Part model, mm, in its own coordinate system. Give positions to 0.01 mm unless a question says otherwise; leave off trailing zeros. Write each loop counter-clockwise with the first axis right and the second up, starting at its lowest first coordinate (ties: lowest second). Pieces come first, ordered by that corner, then holes. Notation, with made-up numbers: M 14,57.25 L 24,57.25 A25 cw 24,91.25 Z; hole C 24,89.25 d11. An arc over 180 degrees is marked long. Answer as CSV lines item,"result". Start each with the question number.
Item 1: Band-saw the part on A-A, the plane y = 8. List the corners of the cut face in (x, z), then the cut area to 3 significant figures.
Item 2: Wall check: L1, parallel to X at y = 0.5, z = 23; L2, parallel to Z at x = 26.5, y = 0; L3, parallel to Z at x = 25, y = 2. Give the ranges that are in metal, low to high. Write a range as from..to.
Item 3: Pin check, flat tips, straight feed: pin 1 (8 mm diameter, centred on y = 0, z = -15, fed in from +X); pin 2 (4 mm diameter, centred on x = -21.5, y = 1, fed in from +Z); pin 3 (5.5 mm diameter, centred on y = 0.5, z = 17.5, fed in from -X). Stop position of each tip, or through.
Item 4: Band-saw the part on B-B, the plane y = 12.5. List the corners of the cut face in (x, z), then the cut area to 3 significant figures.
Item 5: Band-saw the part on C-C, the plane z = 29.5. Count the separate pieces of the cut face and the enclosed holes in it, then the cut area to 3 significant figures.
from build123d import *

# Parameters (mm, degrees)
REVOLVE1_ANGLE                 = 90
BOSS_EXTRUDE2_DEPTH            = 22.5
CUT_EXTRUDE1_DEPTH             = 57.762672959
MIRROR3_START                  = -2.736132077
MIRROR3_DEPTH                  = 5
MIRROR3_START_2                = 2.263867923
MIRROR3_2_DEPTH                = 20.236132077
MIRROR3_3_DEPTH                = 1
MIRROR3_START_3                = 1.263867923
MIRROR3_4_DEPTH                = 1
MIRROR4_START                  = -2.736132077
MIRROR4_DEPTH                  = 5
MIRROR4_START_2                = 2.263867923
MIRROR4_2_DEPTH                = 20.236132077
MIRROR4_3_DEPTH                = 1
MIRROR4_START_3                = 1.263867923
MIRROR4_4_DEPTH                = 1
SKETCH7_R                      = 3.35
CUT_EXTRUDE2_DEPTH             = 20
FILLET9_R                      = 0.5
CUT_EXTRUDE3_REACH             = 59.609
SKETCH8_R                      = 1.5
CUT_EXTRUDE3_DIRECTION_2_REACH = 59.609


# Read off the part's stored shape, not the designer's step: Mirror3, Mirror4
with BuildPart() as part:
    # Sketch1 → Revolve1 (revolve)
    with BuildSketch(Plane.XY):
        Polygon((0, 2.263867923), (0, -2.736132077), (37.5, -2.736132077), (37.5, -1.736132077), (37.25, -1.736132077), (37.25, 1.263867923), (37.5, 1.263867923), (37.5, 2.263867923), align=None)
    revolve(axis=Axis((0, 2.263867923, 0), (0, -1, 0)), revolution_arc=REVOLVE1_ANGLE)

    # Sketch2 → Boss-Extrude2 (add)
    with BuildSketch(Plane(origin=(0, 0, 0), x_dir=(1, 0, 0), z_dir=(0, 1, 0))):
        with BuildLine():
            Line((0, 0), (6, 0))
            ThreePointArc((6, 0), (4.242640687, -4.242640687), (0, -6))
            Line((0, -6), (0, 0))
        make_face()
    extrude(amount=BOSS_EXTRUDE2_DEPTH)

    # Sketch6 → Cut-Extrude1 (cut, through all)
    with BuildSketch(Plane(origin=(0, 2.263867923, 0), x_dir=(1, 0, 0), z_dir=(0, 1, 0))):
        with BuildLine():
            Line((1.75, -5.739120142), (1.75, -32.452850414))
            ThreePointArc((1.75, -32.452850414), (22.980970389, -22.980970389), (32.452850414, -1.75))
            Line((32.452850414, -1.75), (5.739120142, -1.75))
            ThreePointArc((5.739120142, -1.75), (4.242640687, -4.242640687), (1.75, -5.739120142))
        make_face()
    extrude(amount=-CUT_EXTRUDE1_DEPTH, mode=Mode.SUBTRACT)

    # Mirror3 outline → Mirror3 (add)
    with BuildSketch(Plane(origin=(0, 0, 0), x_dir=(1, 0, 0), z_dir=(0, 1, 0)).offset(MIRROR3_START)):
        with BuildLine():
            ThreePointArc((37.25, 0), (26.339727599, 26.339727599), (0, 37.25))
            Line((0, 37.25), (0, 0))
            Line((0, 0), (37.25, 0))
        make_face()
        with BuildLine():
            Line((32.452850414, 1.75), (5.739120142, 1.75))
            ThreePointArc((5.739120142, 1.75), (4.242640687, 4.242640687), (1.75, 5.739120142))
            Line((1.75, 5.739120142), (1.75, 32.452850414))
            ThreePointArc((1.75, 32.452850414), (22.980970389, 22.980970389), (32.452850414, 1.75))
        make_face(mode=Mode.SUBTRACT)
    extrude(amount=MIRROR3_DEPTH)

    # Mirror3 2 outline → Mirror3 2 (add)
    with BuildSketch(Plane(origin=(0, 0, 0), x_dir=(1, 0, 0), z_dir=(0, 1, 0)).offset(MIRROR3_START_2)):
        with BuildLine():
            Line((0, 0), (6, 0))
            ThreePointArc((6, 0), (4.242640687, 4.242640687), (0, 6))
            Line((0, 6), (0, 0))
        make_face()
    extrude(amount=MIRROR3_2_DEPTH)

    # Mirror3 3 outline → Mirror3 3 (add)
    with BuildSketch(Plane(origin=(0, 0, 0), x_dir=(1, 0, 0), z_dir=(0, 1, 0)).offset(MIRROR3_START)):
        with BuildLine():
            Line((37.25, 0), (37.5, 0))
            ThreePointArc((37.5, 0), (26.516504294, 26.516504294), (0, 37.5))
            Line((0, 37.5), (0, 37.25))
            ThreePointArc((0, 37.25), (26.339727599, 26.339727599), (37.25, 0))
        make_face()
    extrude(amount=MIRROR3_3_DEPTH)

    # Mirror3 4 outline → Mirror3 4 (add)
    with BuildSketch(Plane(origin=(0, 0, 0), x_dir=(1, 0, 0), z_dir=(0, 1, 0)).offset(MIRROR3_START_3)):
        with BuildLine():
            Line((37.25, 0), (37.5, 0))
            ThreePointArc((37.5, 0), (26.516504294, 26.516504294), (0, 37.5))
            Line((0, 37.5), (0, 37.25))
            ThreePointArc((0, 37.25), (26.339727599, 26.339727599), (37.25, 0))
        make_face()
    extrude(amount=MIRROR3_4_DEPTH)

    # Mirror4 outline → Mirror4 (add)
    with BuildSketch(Plane(origin=(0, 0, 0), x_dir=(1, 0, 0), z_dir=(0, 1, 0)).offset(MIRROR4_START)):
        with BuildLine():
            ThreePointArc((0, 37.25), (-37.25, 0), (0, -37.25))
            Line((0, -37.25), (0, 37.25))
        make_face()
        with BuildLine():
            Line((-1.75, 32.452850414), (-1.75, 5.739120142))
            ThreePointArc((-1.75, 5.739120142), (-4.242640687, 4.242640687), (-5.739120142, 1.75))
            Line((-5.739120142, 1.75), (-32.452850414, 1.75))
            ThreePointArc((-32.452850414, 1.75), (-22.980970389, 22.980970389), (-1.75, 32.452850414))
        make_face(mode=Mode.SUBTRACT)
        with BuildLine():
            Line((-32.452850414, -1.75), (-5.739120142, -1.75))
            ThreePointArc((-5.739120142, -1.75), (-4.242640687, -4.242640687), (-1.75, -5.739120142))
            Line((-1.75, -5.739120142), (-1.75, -32.452850414))
            ThreePointArc((-1.75, -32.452850414), (-22.980970389, -22.980970389), (-32.452850414, -1.75))
        make_face(mode=Mode.SUBTRACT)
    extrude(amount=MIRROR4_DEPTH)

    # Mirror4 2 outline → Mirror4 2 (add)
    with BuildSketch(Plane(origin=(0, 0, 0), x_dir=(1, 0, 0), z_dir=(0, 1, 0)).offset(MIRROR4_START_2)):
        with BuildLine():
            Line((0, -6), (0, 6))
            ThreePointArc((0, 6), (-6, 0), (0, -6))
        make_face()
    extrude(amount=MIRROR4_2_DEPTH)

    # Mirror4 3 outline → Mirror4 3 (add)
    with BuildSketch(Plane(origin=(0, 0, 0), x_dir=(1, 0, 0), z_dir=(0, 1, 0)).offset(MIRROR4_START)):
        with BuildLine():
            Line((0, 37.25), (0, 37.5))
            ThreePointArc((0, 37.5), (-37.5, 0), (0, -37.5))
            Line((0, -37.5), (0, -37.25))
            ThreePointArc((0, -37.25), (-37.25, 0), (0, 37.25))
        make_face()
    extrude(amount=MIRROR4_3_DEPTH)

    # Mirror4 4 outline → Mirror4 4 (add)
    with BuildSketch(Plane(origin=(0, 0, 0), x_dir=(1, 0, 0), z_dir=(0, 1, 0)).offset(MIRROR4_START_3)):
        with BuildLine():
            Line((0, 37.25), (0, 37.5))
            ThreePointArc((0, 37.5), (-37.5, 0), (0, -37.5))
            Line((0, -37.5), (0, -37.25))
            ThreePointArc((0, -37.25), (-37.25, 0), (0, 37.25))
        make_face()
    extrude(amount=MIRROR4_4_DEPTH)

    # Sketch7 → Cut-Extrude2 (cut)
    with BuildSketch(Plane(origin=(0, 22.5, 0), x_dir=(1, 0, 0), z_dir=(0, 1, 0))):
        with Locations(Location((0, 0, 0), (0, 0, 270))):
            Circle(SKETCH7_R)
    extrude(amount=-CUT_EXTRUDE2_DEPTH, mode=Mode.SUBTRACT)

    # Fillet9
    # the kernel refuses this fillet: 0.5 mm, written as the material it adds along each edge
    with BuildSketch(Plane(origin=(0, 1.263867923, 0), x_dir=(0, 0, 1), z_dir=(1, 0, 0))) as fillet9_piece_1:
        with BuildLine():
            CenterArc((37.75, 0.433012702), FILLET9_R, 180, 60)
            Line((37.5, 0), (37.495, -0.008660254))
            ThreePointArc((37.495, -0.008660254), (37.375, -0.01), (37.25, -0.01))
            Line((37.25, -0.01), (37.24, 0))
            Line((37.24, 0), (37.24, 0.433012702))
            Line((37.24, 0.433012702), (37.25, 0.433012702))
        make_face()
    revolve(axis=Axis((0, 1.263867923, 0), (0, -1, 0)), revolution_arc=180)
    with BuildSketch(Plane(origin=(0, -1.736132077, 0), x_dir=(0, 0, 1), z_dir=(1, 0, 0))) as fillet9_piece_2:
        with BuildLine():
            CenterArc((37.75, -0.433012702), FILLET9_R, 120, 60)
            Line((37.25, -0.433012702), (37.24, -0.433012702))
            Line((37.24, -0.433012702), (37.24, 0))
            Line((37.24, 0), (37.25, 0.01))
            ThreePointArc((37.25, 0.01), (37.375, 0.01), (37.495, 0.008660254))
            Line((37.495, 0.008660254), (37.5, 0))
        make_face()
    revolve(axis=Axis((0, -1.736132077, 0), (0, -1, 0)), revolution_arc=180)
    with BuildSketch(Plane(origin=(0, -1.736132077, 0), x_dir=(1, 0, 0), z_dir=(0, 0, -1))) as fillet9_piece_3:
        with BuildLine():
            CenterArc((37.75, -0.433012702), FILLET9_R, 120, 60)
            Line((37.25, -0.433012702), (37.24, -0.433012702))
            Line((37.24, -0.433012702), (37.24, 0))
            Line((37.24, 0), (37.25, 0.01))
            ThreePointArc((37.25, 0.01), (37.375, 0.01), (37.495, 0.008660254))
            Line((37.495, 0.008660254), (37.5, 0))
        make_face()
    revolve(axis=Axis((0, -1.736132077, 0), (0, -1, 0)), revolution_arc=90)
    with BuildSketch(Plane(origin=(-1e-09, -1.736132077, 1e-09), x_dir=(1.823040450855093e-11, 0, -1.0), z_dir=(-1.0, 0, -1.823040450855093e-11))) as fillet9_piece_4:
        with BuildLine():
            CenterArc((37.750000001, -0.433012702), FILLET9_R, 120, 60)
            Line((37.250000001, -0.433012702), (37.240000001, -0.433012702))
            Line((37.240000001, -0.433012702), (37.240000001, 0))
            Line((37.240000001, 0), (37.250000001, 0.01))
            ThreePointArc((37.250000001, 0.01), (37.375000001, 0.01), (37.495000001, 0.008660254))
            Line((37.495000001, 0.008660254), (37.500000001, 0))
        make_face()
    revolve(axis=Axis((-1e-09, -1.736132077, 1e-09), (0, -1, 0)), revolution_arc=89.999999998)
    with BuildSketch(Plane(origin=(0, 1.263867923, 0), x_dir=(1, 0, 0), z_dir=(0, 0, -1))) as fillet9_piece_5:
        with BuildLine():
            CenterArc((37.75, 0.433012702), FILLET9_R, 180, 60)
            Line((37.5, 0), (37.495, -0.008660254))
            ThreePointArc((37.495, -0.008660254), (37.375, -0.01), (37.25, -0.01))
            Line((37.25, -0.01), (37.24, 0))
            Line((37.24, 0), (37.24, 0.433012702))
            Line((37.24, 0.433012702), (37.25, 0.433012702))
        make_face()
    revolve(axis=Axis((0, 1.263867923, 0), (0, -1, 0)), revolution_arc=90)
    with BuildSketch(Plane(origin=(-1e-09, 1.263867923, 1e-09), x_dir=(1.823040450855093e-11, 0, -1.0), z_dir=(-1.0, 0, -1.823040450855093e-11))) as fillet9_piece_6:
        with BuildLine():
            CenterArc((37.750000001, 0.433012702), FILLET9_R, 180, 60)
            Line((37.500000001, 0), (37.495000001, -0.008660254))
            ThreePointArc((37.495000001, -0.008660254), (37.375000001, -0.01), (37.250000001, -0.01))
            Line((37.250000001, -0.01), (37.240000001, 0))
            Line((37.240000001, 0), (37.240000001, 0.433012702))
            Line((37.240000001, 0.433012702), (37.250000001, 0.433012702))
        make_face()
    revolve(axis=Axis((-1e-09, 1.263867923, 1e-09), (0, -1, 0)), revolution_arc=89.999999998)

    # Sketch8 → Cut-Extrude3 (cut, up to next)
    with BuildSketch(Plane.XY, mode=Mode.PRIVATE) as cut_extrude3_sk1:
        with Locations((0, 12.5)):
            Circle(SKETCH8_R)
    cut_extrude3_tool1 = extrude(cut_extrude3_sk1.sketch, amount=-CUT_EXTRUDE3_REACH, mode=Mode.PRIVATE) & part.part
    add(cut_extrude3_tool1.solids().sort_by_distance((0, 12.5, 0))[0], mode=Mode.SUBTRACT)

    # Sketch8 → Cut-Extrude3 direction 2 (cut, up to next)
    with BuildSketch(Plane.XY, mode=Mode.PRIVATE) as cut_extrude3_direction_2_sk1:
        with Locations((0, 12.5)):
            Circle(SKETCH8_R)
    cut_extrude3_direction_2_tool1 = extrude(cut_extrude3_direction_2_sk1.sketch, amount=CUT_EXTRUDE3_DIRECTION_2_REACH, mode=Mode.PRIVATE) & part.part
    add(cut_extrude3_direction_2_tool1.solids().sort_by_distance((0, 12.5, 0))[0], mode=Mode.SUBTRACT)


solid = part.part
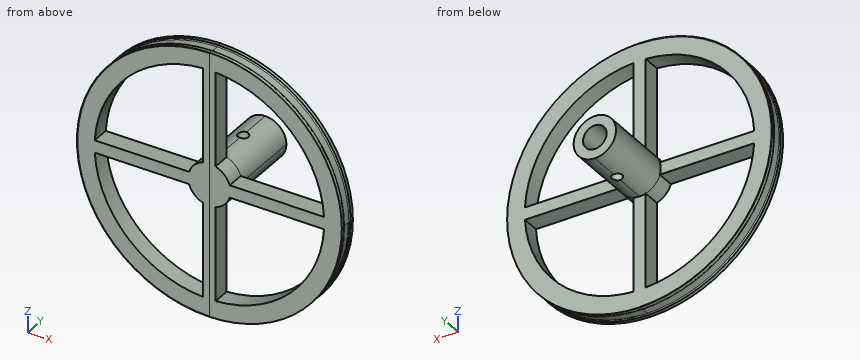
Output:
1,outline,"C 0,0 d12; hole C 0,0 d6.7"
1,area,"77.8 mm²"
2,L1,"-29.3..-22.96, -1.75..1.75, 22.96..29.3"
2,L2,"-26.18..-18.81, -1.75..1.75, 18.81..26.18"
2,L3,"-27.95..-20.77, -1.75..1.75, 20.77..27.95"
3,pin 1,"x = 35.79"
3,pin 2,"z = 32.02"
3,pin 3,"x = -34.43"
4,outline,"M -1.5,-5.81 L -1.5,-3 A3.35 cw -1.5,3 L -1.5,5.81 A6 ccw Z; M 1.5,-5.81 A6 ccw 1.5,5.81 L 1.5,3 A3.35 cw 1.5,-3 Z"
4,area,"61.6 mm²"
5,separate pieces,"3"
5,enclosed holes,"0"
5,area,"110 mm²"
